For this review, take the finished solid that the model builds, in its own axes (mm). Round coordinates to 2 decimals unless told otherwise and drop trailing zeros. Write each loop counter-clockwise with the first axis right and the second up, starting at its lowest first coordinate (ties: lowest second). Pieces come first, ordered by that corner, then holes. Notation, with made-up numbers: (-35, 12.25) -> (23, 12.25) arc R21 cw to (23, 47.25) -> close; hole circle Ø11 at (2.25, 9.25). An arc over 180 degrees is marked (long way). Answer in a Markdown table with one row per item.
from build123d import *

# Parameters (mm, degrees)
SKETCH1_R           = 0.9
BOSS_EXTRUDE1_DEPTH = 6
SKETCH7_R           = 0.125
SKETCH8_R           = 0.125


with BuildPart() as part:
    # Sketch1 → Boss-Extrude1 (new body)
    with BuildSketch(Plane(origin=(0, 0, 0), x_dir=(1, 0, 0), z_dir=(0, 1, 0))):
        with Locations(Location((0, 0, 0), (0, 0, 270))):
            Circle(SKETCH1_R)
    extrude(amount=BOSS_EXTRUDE1_DEPTH)

    # Sweep1: sweep along a path in Sketch4
    with BuildLine() as sweep1_path:  # in the path sketch's own coordinates; laid on its plane below (add() does not lay a ready-made edge on the line's plane)
        add(Edge.make_bspline(
            [(0, -0.355), (2.024905843, -0.343321446), (0.641829723, -1.574292855), (3, -1.578751128)],
            knots=[0, 0, 0, 0, 1, 1, 1, 1], degree=3))
    # Sketch7 → Sweep1 (sweep)
    with BuildSketch(Plane.XZ):
        with Locations((-0.502045815, 0)):
            Circle(SKETCH7_R)
    sweep(path=Plane(origin=(-0.251022907, 0, 0.251022907), x_dir=(0, -1, 0), z_dir=(-0.7071067811865488, 0, 0.7071067811865464)) * sweep1_path.line)

    # Sweep2: sweep along a path in Sketch6
    with BuildLine() as sweep2_path:  # in the path sketch's own coordinates; laid on its plane below (add() does not lay a ready-made edge on the line's plane)
        add(Edge.make_bspline(
            [(0, -0.355), (2.024905843, -0.343321446), (0.641829723, -1.568079226), (3, -1.572537499)],
            knots=[0, 0, 0, 0, 1, 1, 1, 1], degree=3))
    # Sketch8 → Sweep2 (sweep)
    with BuildSketch(Plane.XZ):
        with Locations((0.502045815, 0)):
            Circle(SKETCH8_R)
    sweep(path=Plane(origin=(0.251022907, 0, 0.251022907), x_dir=(0, -1, 0), z_dir=(-0.7071067811865464, 0, -0.7071067811865488)) * sweep2_path.line)


solid = part.part
1) For line 1 (Y direction, x = -0.5, z = 0.25); line 2 (X direction, y = -2.25, z = -0.85); line 3 (Z direction, x = 0.05, y = 3), list the stretches that pass through material, from the lowest coordinate up. Write a range as [from, to].
Solved:
| item | result |
|---|---|
| line 1 | [0, 6] |
| line 2 | [-1.45, -1.2], [1.2, 1.44] |
| line 3 | [-0.9, 0.9] |
2) Consider section B-B on y = 2.75. State the section outline as (x, z) points.
Solved:
| item | result |
|---|---|
| outline | circle Ø1.8 at (0, 0) |
3) Clearance check with flat-ended pins moving along their axes: pin 1 Ø1 at (y, z) = (0, -0.5) entering from +X; pin 2 Ø1 at (x, y) = (-0.5, -1) entering from -Z. State where each tip first meets the part, or that it passes through.
Solved:
| item | result |
|---|---|
| pin 1 | x = 0.9 |
| pin 2 | z = -0.53 |
4) Consider section A-A on x = 0. State the section outline as (y, z) points.
Solved:
| item | result |
|---|---|
| outline | (0, -0.9) -> (6, -0.9) -> (6, 0.9) -> (0, 0.9) -> close |
5) Consider section C-C on z = 0.75. State the section outline as (x, y) points.
Solved:
| item | result |
|---|---|
| outline | (-0.5, 0) -> (0.5, 0) -> (0.5, 6) -> (-0.5, 6) -> close |
